Check sheet for the modelled part. Datum: model origin and axes. Units: mm. A direction names the side the tool comes from. Coordinates: 2 decimals unless noted, no trailing zeros. Loops run counter-clockwise (first coordinate to the right, second up) from the corner with the lowest first, then second, coordinate; pieces in that order, holes last. Notation, with made-up numbers: (31.25, 55) -> (84.25, 55) arc R22 ccw to (84.25, 73) -> close; hole circle Ø4 at (46, -28.5). An arc over 180 degrees is marked (long way). Use CSV: the item, a comma, the result in double quotes. Start each with the question number.
1. Sectioned sample at C-C, the plane z = 0.15. Record the cut outline in (x, y).
2. Sectioned sample at B-B, the plane y = 2.05. Record the cut outline in (x, z), and give its area (3 significant figures).
3. Sectioned sample at A-A, the plane x = -2.5. Record the cut outline in (y, z).
4. Release check for a two-part mould opening along X. For faces 1 (the face through (-6.487, 4.641, 1.972)), 2 (the face through (0, 2.4, -0.3)), 3 (the face through (-1.72, 0.54, -0.99)), 4 (the face through (-5.6, -0.5, 4)) record: pulls with the +X half, pulls with the -X half, needs draft (parallel to the pull), parting line crosses it, or undercut.
5. Thickness scan on L1, parallel to Y at x = -2.5, z = -1.55; L2, parallel to Y at x = -4.75, z = 1.5; L3, parallel to Z at x = -6.5, y = 1.75. Record the ranges inside material, lowest first.
6. Set-up check for faces 5 (the face through (-4, 5, 4)), 6 (the face through (-6, 0, 2)), 7 (the face through (-7, 2, 0)): record each of +Z, -Z, +X, -X, +Y, -Y from which the full face is reachable in a straight line by a thin tool's end or side.
7. Sectioned sample at D-D, the plane x = -5.5. Record the cut outline in (y, z).
```python
from build123d import *

# Parameters (mm, degrees)
BOSS_EXTRUDE1_DEPTH   = 4
SKETCH2_W             = 11
SKETCH2_H             = 1
BOSS_EXTRUDE1_2_DEPTH = 4
SKETCH3_W             = 11
SKETCH3_H             = 6.9
BOSS_EXTRUDE2_DEPTH   = 2
SKETCH5_R             = 1.7
CUT_EXTRUDE1_DEPTH    = 2


with BuildPart() as part:
    # Sketch2 → Boss-Extrude1 (new body)
    with BuildSketch(Plane.XY):
        with BuildLine():
            Line((-5, 4.1), (0, 4.1))
            Line((0, 4.1), (0, 5.1))
            Line((0, 5.1), (0, 5.9))
            Line((0, 5.9), (-5, 5.9))
            Line((-5, 5.9), (-7, 5.9))
            ThreePointArc((-7, 5.9), (-6.472792206, 4.627207794), (-5.2, 4.1))
            Line((-5.2, 4.1), (-5, 4.1))
        make_face()
    extrude(amount=BOSS_EXTRUDE1_DEPTH)



with BuildPart() as body_2:
    # Sketch2 → Boss-Extrude1 2 (new body)
    with BuildSketch(Plane.XY):
        with Locations((-5.5, -0.5)):
            Rectangle(SKETCH2_W, SKETCH2_H)
    extrude(amount=BOSS_EXTRUDE1_2_DEPTH)


with BuildPart() as part_1:
    add(part.part)

    add(body_2.part)  # Boss-Extrude2 merges body 2
    # Sketch3 → Boss-Extrude2 (add)
    with BuildSketch(Plane(origin=(0, 0, 0), x_dir=(-1, 0, 0), z_dir=(0, 0, -1))):
        with Locations((5.5, 2.45)):
            Rectangle(SKETCH3_W, SKETCH3_H)
    extrude(amount=BOSS_EXTRUDE2_DEPTH)

    # Sketch5 → Cut-Extrude1 (cut)
    with BuildSketch(Plane.XY):
        with Locations((-2.5, 2.05)):
            Circle(SKETCH5_R)
    extrude(amount=-CUT_EXTRUDE1_DEPTH, mode=Mode.SUBTRACT)


solid = part_1.part
```
Completed:
1,outline,"(-11, -1) -> (0, -1) -> (0, 0) -> (-11, 0) -> close; (-7, 5.9) arc R1.8 ccw to (-5.2, 4.1) -> (0, 4.1) -> (0, 5.9) -> close"
2,outline,"(-11, -2) -> (-4.2, -2) -> (-4.2, 0) -> (-11, 0) -> close; (-0.8, -2) -> (0, -2) -> (0, 0) -> (-0.8, 0) -> close"
2,area,"15.2 mm²"
3,outline,"(-1, -2) -> (0.35, -2) -> (0.35, 0) -> (0, 0) -> (0, 4) -> (-1, 4) -> close; (3.75, -2) -> (5.9, -2) -> (5.9, 4) -> (4.1, 4) -> (4.1, 0) -> (3.75, 0) -> close"
4,face 1,"pulls with the -X half"
4,face 2,"pulls with the +X half"
4,face 3,"undercut"
4,face 4,"needs draft"
5,L1,"-1 to 0.35, 3.75 to 5.9"
5,L2,"-1 to 0, 4.1 to 5.9"
5,L3,"-2 to 0"
6,face 5,"+Z, +X, -X, +Y, -Y"
6,face 6,"+Z, +X, -X"
6,face 7,"+Z, -X"
7,outline,"(-1, -2) -> (5.9, -2) -> (5.9, 4) -> (4.13, 4) -> (4.13, 0) -> (0, 0) -> (0, 4) -> (-1, 4) -> close"
